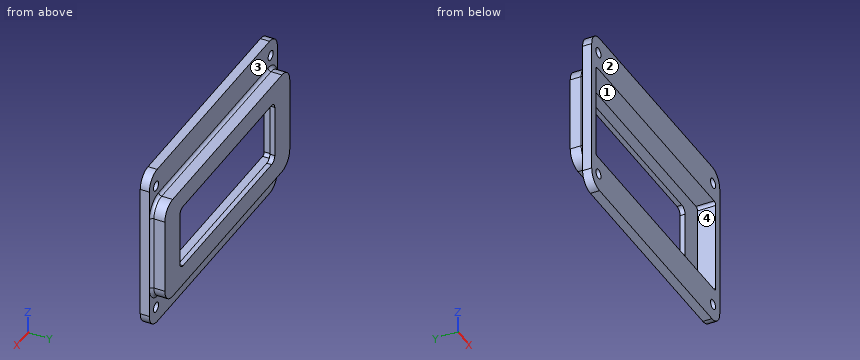
from build123d import *

# Parameters (mm, degrees)
SKETCH1_W           = 104.14
SKETCH1_H           = 69.85
BOSS_EXTRUDE1_DEPTH = 3.81
SKETCH2_W           = 101.6
SKETCH2_H           = 44.45
BOSS_EXTRUDE2_DEPTH = 5.842
SKETCH4_W           = 97.536
SKETCH4_H           = 40.64
CUT_EXTRUDE1_DEPTH  = 7.62
SKETCH5_W           = 77.216
SKETCH5_H           = 27.178
CUT_EXTRUDE2_DEPTH  = 5.842
FILLET1_R           = 2.54
FILLET2_R           = 6.35
FILLET3_R           = 1.27
SKETCH6_R           = 2.032
CUT_EXTRUDE3_DEPTH  = 5.842
FILLET4_R           = 1.27


with BuildPart() as part:
    # Sketch1 → Boss-Extrude1 (new body)
    with BuildSketch(Plane(origin=(0, 0, 0), x_dir=(1, 0, 0), z_dir=(0, 1, 0))):
        Rectangle(SKETCH1_W, SKETCH1_H)
    extrude(amount=BOSS_EXTRUDE1_DEPTH)

    # Sketch2 → Boss-Extrude2 (add)
    with BuildSketch(Plane(origin=(0, 3.81, 0), x_dir=(1, 0, 0), z_dir=(0, 1, 0))):
        Rectangle(SKETCH2_W, SKETCH2_H)
    extrude(amount=BOSS_EXTRUDE2_DEPTH)

    # Sketch4 → Cut-Extrude1 (cut)
    with BuildSketch(Plane.XZ):
        Rectangle(SKETCH4_W, SKETCH4_H)
    extrude(amount=-CUT_EXTRUDE1_DEPTH, mode=Mode.SUBTRACT)

    # Sketch5 → Cut-Extrude2 (cut)
    with BuildSketch(Plane.XZ.offset(-7.62)):
        Rectangle(SKETCH5_W, SKETCH5_H)
    extrude(amount=-CUT_EXTRUDE2_DEPTH, mode=Mode.SUBTRACT)

    # Fillet1
    fillet1_edges = [part.edges().sort_by_distance(p)[0] for p in [
        (-38.608, 8.636, -13.589),
        (-38.608, 8.636, 13.589),
        (38.608, 8.636, 13.589),
        (38.608, 8.636, -13.589),
    ]]
    fillet(fillet1_edges, radius=FILLET1_R)

    # Fillet2
    fillet2_edges = [part.edges().sort_by_distance(p)[0] for p in [
        (50.8, 6.731, 22.225),
        (50.8, 6.731, -22.225),
        (-50.8, 6.731, -22.225),
        (-50.8, 6.731, 22.225),
        (-52.07, 1.905, -34.925),
        (52.07, 1.905, -34.925),
        (52.07, 1.905, 34.925),
        (-52.07, 1.905, 34.925),
    ]]
    fillet(fillet2_edges, radius=FILLET2_R)

    # Fillet3
    fillet3_edges = [part.edges().sort_by_distance(p)[0] for p in [
        (0, 3.81, -22.225),
        (50.8, 3.81, 0),
        (0, 3.81, 22.225),
        (-50.8, 3.81, 0),
        (48.940128061, 3.81, -20.365128061),
        (-48.940128061, 3.81, -20.365128061),
        (-48.940128061, 3.81, 20.365128061),
        (48.940128061, 3.81, 20.365128061),
    ]]
    fillet(fillet3_edges, radius=FILLET3_R - 0.0001)  # a hair under: the kernel refuses the full size

    # Sketch6 → Cut-Extrude3 (cut)
    with BuildSketch(Plane(origin=(0, 3.81, 0), x_dir=(1, 0, 0), z_dir=(0, 1, 0))):
        with Locations(Location((-46.609, 27.84475, 0), (0, 0, 270))):
            Circle(SKETCH6_R)
        with Locations(Location((46.609, 27.84475, 0), (0, 0, 270))):
            Circle(SKETCH6_R)
        with Locations(Location((46.609, -27.84475, 0), (0, 0, 270))):
            Circle(SKETCH6_R)
        with Locations(Location((-46.609, -27.84475, 0), (0, 0, 270))):
            Circle(SKETCH6_R)
    extrude(amount=-CUT_EXTRUDE3_DEPTH, mode=Mode.SUBTRACT)

    # Fillet4
    fillet4_edges = [part.edges().sort_by_distance(p)[0] for p in [
        (-48.768, 3.81, -20.32),
        (-48.768, 3.81, 20.32),
        (48.768, 3.81, 20.32),
        (48.768, 3.81, -20.32),
    ]]
    fillet(fillet4_edges, radius=FILLET4_R)


solid = part.part
Read the model definition and answer for the solid it produces. Units are mm, in the model's axes. Face numbers are marked on the shaded views. A direction names the side the tool comes from. Round coordinates to 2 decimals unless told otherwise and drop trailing zeros. Write each loop counter-clockwise with the first axis right and the second up, starting at its lowest first coordinate (ties: lowest second). Pieces come first, ordered by that corner, then holes. Notation, with made-up numbers: M -2.5,-19 L 22.5,-19 A13 ccw 22.5,-9 Z; hole C 46,73 d6. An arc over 180 degrees is marked long. Use a Markdown table: item, result.
1) Straight lines are drawn through the part: line 1 along X through (y, z) = (5.5, -1.5); line 2 along X through (y, z) = (2.5, 6.5); line 3 along Z through (x, y) = (-33.5, 9.25) (3 decimals). For each, find the intervals that lie inside material, in ascending order. Write a range as [from, to].
Answers follow:
| item | result |
|---|---|
| line 1 | x = [-50.8, -48.77], [48.77, 50.8] |
| line 2 | x = [-52.07, -48.77], [48.77, 52.07] |
| line 3 | z = [-22.225, -13.589], [13.589, 22.225] |
2) For a pull along X with two mould halves and no side action, classify the marked faces 3 and 4 as pulls with the +X half, pulls with the -X half, needs draft (parallel to the pull), parting line crosses it, or undercut.
Answers follow:
| item | result |
|---|---|
| face 3 | needs draft |
| face 4 | undercut |
3) Flat-ended cylindrical pins translate along their axes: pin 1 (1.6 mm diameter, centred on y = 9, z = -1.5, fed in from +X); pin 2 (1.6 mm diameter, centred on y = 8.5, z = -0.5, fed in from -X); pin 3 (5.5 mm diameter, centred on x = -46.61, z = 27.84, fed in from +Y). Find the tip coordinate at first contact, or state that the pin passes through.
Answers follow:
| item | result |
|---|---|
| pin 1 | stops at x = 50.8 |
| pin 2 | stops at x = -50.8 |
| pin 3 | stops at y = 3.81 |
4) The part is cut by section A-A (x = -9). Write down the section's boundary in (y, z) (3 decimals).
Answers follow:
| item | result |
|---|---|
| outline | M 0,-34.925 L 3.81,-34.925 L 3.81,-23.495 A1.27 cw 5.08,-22.225 L 9.652,-22.225 L 9.652,-13.589 L 7.62,-13.589 L 7.62,-20.32 L 0,-20.32 Z; M 0,20.32 L 7.62,20.32 L 7.62,13.589 L 9.652,13.589 L 9.652,22.225 L 5.08,22.225 A1.27 cw 3.81,23.495 L 3.81,34.925 L 0,34.925 Z |
5) The part is cut by section C-C (z = 27). Write down the section's boundary in (x, y), plus the area to 3 significant figures.
Answers follow:
| item | result |
|---|---|
| outline | M -52.07,0 L -48.46,0 L -48.46,3.81 L -52.07,3.81 Z; M -44.76,0 L 44.76,0 L 44.76,3.81 L -44.76,3.81 Z; M 48.46,0 L 52.07,0 L 52.07,3.81 L 48.46,3.81 Z |
| area | 369 mm2 |
6) The part is cut by section D-D (y = 1.5). Write down the section's boundary in (x, z) (3 decimals).
Answers follow:
| item | result |
|---|---|
| outline | M -52.07,-28.575 A6.35 ccw -45.72,-34.925 L 45.72,-34.925 A6.35 ccw 52.07,-28.575 L 52.07,28.575 A6.35 ccw 45.72,34.925 L -45.72,34.925 A6.35 ccw -52.07,28.575 Z; hole M -48.768,-19.05 A1.27 ccw -47.498,-20.32 L 47.498,-20.32 A1.27 ccw 48.768,-19.05 L 48.768,19.05 A1.27 ccw 47.498,20.32 L -47.498,20.32 A1.27 ccw -48.768,19.05 Z; hole C -46.609,-27.845 d4.064; hole C -46.609,27.845 d4.064; hole C 46.609,-27.845 d4.064; hole C 46.609,27.845 d4.064 |
7) A tool of negligible diameter and unlimited length cuts with its end or side. For the marked faces 1 and 2, from which of +Z, -Z, +X, -X, +Y, -Y can it reach the whole face along a straight path? Write none if from no direction.
Answers follow:
| item | result |
|---|---|
| face 1 | -Y |
| face 2 | +Z, -Z, +X, -X, -Y |
